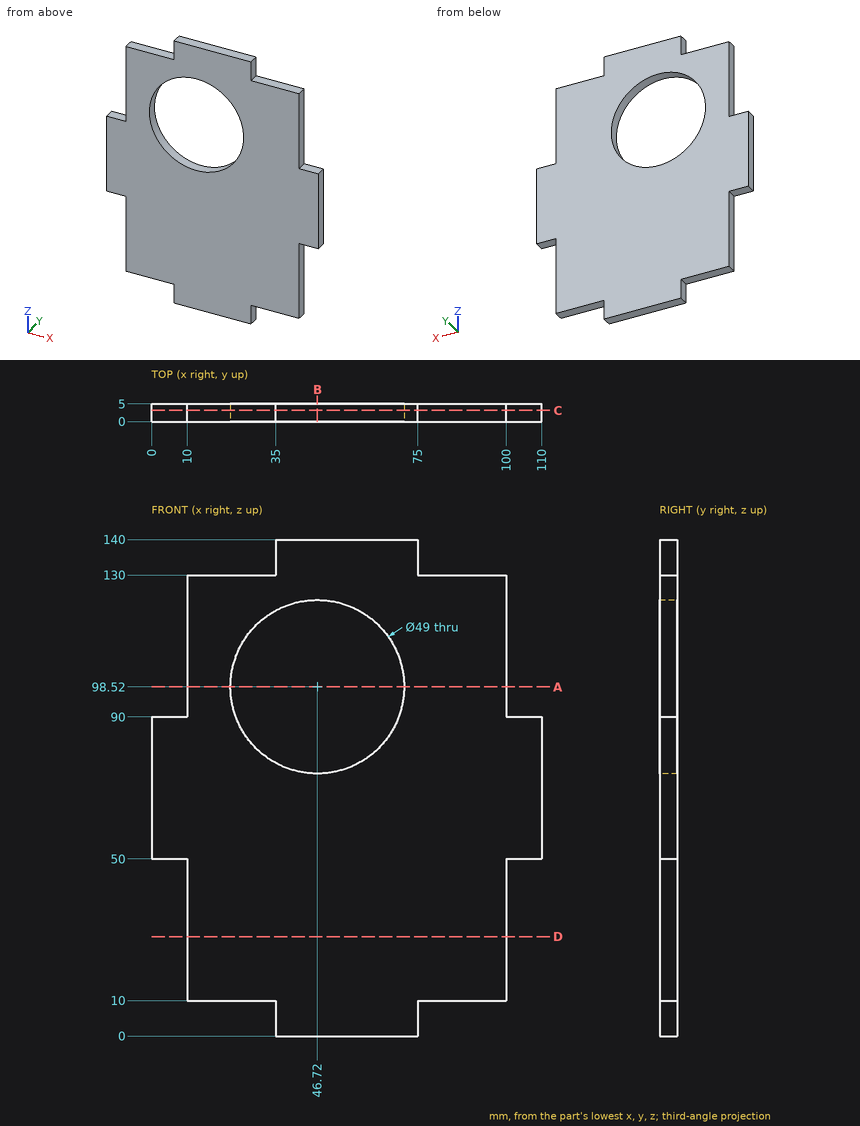
Input: dimensioned drawing with shaded views. Units: mm. Origin: part minimum x, y, z. Give positions to 0.01 mm unless a question says otherwise; leave off trailing zeros. Write each loop counter-clockwise with the first axis right and the second up, starting at its lowest first coordinate (ties: lowest second). Pieces come first, ordered by that corner, then holes. Notation, with made-up numbers: M -3,89.5 L 50,89.5 A26 ccw 50,124.5 Z; hole C 16.5,67 d7. An arc over 180 degrees is marked long. Return JSON: item names as keys, results as strings. Group by question number.
1) Cut plane D-D, the plane z = 28. Output: boundary loops of the cut face in (x, y).
2) Cut plane C-C, the plane y = 3.2. Output: boundary loops of the cut face in (x, z), plus the area to 3 significant figures.
3) Cut plane B-B, the plane x = 46.72. Output: boundary loops of the cut face in (y, z), plus the area to 3 significant figures.
4) Pin query (flat end, axial travel): P1, Ø8, axis at x = 70, z = 99.5, coming from the +Y side; P2, Ø1.5, axis at y = 3, z = 103, coming from the +X side; P3, Ø2.5, axis at y = 3, z = 133.5, coming from the -X side; P4, Ø2, axis at y = 1, z = 33, coming from the -X side. Return the tip coordinate at first contact, or that it passes through.
5) Material intervals for line 1 along X through (y, z) = (2.9, 98.52); line 2 along X through (y, z) = (0.9, 125); line 3 along X through (y, z) = (4.05, 115), sorted ascending. Write a range as [from, to].
6) Cut plane A-A, the plane z = 98.52. Output: boundary loops of the cut face in (x, y).
Recorded:
{
 "1": {"outline": "M 10,0 L 100,0 L 100,5 L 10,5 Z"},
 "2": {"outline": "M 0,50 L 10,50 L 10,10 L 35,10 L 35,0 L 75,0 L 75,10 L 100,10 L 100,50 L 110,50 L 110,90 L 100,90 L 100,130 L 75,130 L 75,140 L 35,140 L 35,130 L 10,130 L 10,90 L 0,90 Z; hole C 46.72,98.52 d49", "area": "10,500 mm²"},
 "3": {"outline": "M 0,0 L 5,0 L 5,74.02 L 0,74.02 Z; M 0,123.02 L 5,123.02 L 5,140 L 0,140 Z", "area": "455 mm²"},
 "4": {"P1": "stops at y = 5", "P2": "stops at x = 100", "P3": "stops at x = 35", "P4": "stops at x = 10"},
 "5": {"line 1": "x = [10, 22.22], [71.22, 100]", "line 2": "x = [10, 100]", "line 3": "x = [10, 28.59], [64.85, 100]"},
 "6": {"outline": "M 10,0 L 22.22,0 L 22.22,5 L 10,5 Z; M 71.22,0 L 100,0 L 100,5 L 71.22,5 Z"}
}
